```python
from build123d import *

# Parameters (mm, degrees)
SKETCH_1_R          = 1
EXTRUDE_1_DEPTH     = 3
FILLET_1_R          = 10
FILLET_2_R          = 10
FILLET_3_R          = 5
FILLET_4_R          = 3
FILLET_5_R          = 10
SKETCH_5_R          = 1.5
CUT_EXTRUDE_2_DEPTH = 10
SKETCH_6_W          = 40
SKETCH_6_H          = 36.981974808
CUT_EXTRUDE_3_DEPTH = 10
FILLET_6_R          = 10
SKETCH_7_R          = 1.5
CUT_EXTRUDE_4_DEPTH = 31


with BuildPart() as part:
    # Sketch 1 → Extrude 1 (new body)
    with BuildSketch(Plane.XY):
        Polygon((0, -15), (0, 15), (41, 15), (49, 67.5), (180.2, 67.5), (180.2, 49.5), (68.511096619, 49.5), (60.968239476, 0), (68.511096619, -49.5), (180.2, -49.5), (180.2, -67.5), (49, -67.5), (41, -15), align=None)
        with Locations((177.2, 54)):
            Circle(SKETCH_1_R, mode=Mode.SUBTRACT)
        with Locations((177.2, 63)):
            Circle(SKETCH_1_R, mode=Mode.SUBTRACT)
        with Locations((177.2, -54)):
            Circle(SKETCH_1_R, mode=Mode.SUBTRACT)
        with Locations((177.2, -63)):
            Circle(SKETCH_1_R, mode=Mode.SUBTRACT)
        with Locations((71, 58.5)):
            Circle(SKETCH_1_R, mode=Mode.SUBTRACT)
        with Locations((54, 58.5)):
            Circle(SKETCH_1_R, mode=Mode.SUBTRACT)
        with Locations((71, -58.5)):
            Circle(SKETCH_1_R, mode=Mode.SUBTRACT)
        with Locations((54, -58.5)):
            Circle(SKETCH_1_R, mode=Mode.SUBTRACT)
        with BuildLine():
            Line((85, -56), (97, -56))
            ThreePointArc((97, -56), (99.5, -58.5), (97, -61))
            Line((97, -61), (85, -61))
            ThreePointArc((85, -61), (82.5, -58.5), (85, -56))
        make_face(mode=Mode.SUBTRACT)
        with BuildLine():
            Line((85, 56), (97, 56))
            ThreePointArc((97, 56), (99.5, 58.5), (97, 61))
            Line((97, 61), (85, 61))
            ThreePointArc((85, 61), (82.5, 58.5), (85, 56))
        make_face(mode=Mode.SUBTRACT)
    extrude(amount=EXTRUDE_1_DEPTH)

    # Fillet 1
    fillet_1_edges = [part.edges().sort_by_distance(p)[0] for p in [
        (41, -15, 1.5),
        (41, 15, 1.5),
    ]]
    fillet(fillet_1_edges, radius=FILLET_1_R)

    # Fillet 2
    fillet_2_edges = [part.edges().sort_by_distance(p)[0] for p in [
        (68.511096619, -49.5, 1.5),
        (68.511096619, 49.5, 1.5),
    ]]
    fillet(fillet_2_edges, radius=FILLET_2_R)

    # Fillet 3
    fillet_3_edges = [part.edges().sort_by_distance(p)[0] for p in [
        (0, -15, 1.5),
        (0, 15, 1.5),
    ]]
    fillet(fillet_3_edges, radius=FILLET_3_R)

    # Fillet 4
    fillet_4_edges = [part.edges().sort_by_distance(p)[0] for p in [
        (180.2, -49.5, 1.5),
        (180.2, -67.5, 1.5),
        (49, -67.5, 1.5),
        (49, 67.5, 1.5),
        (180.2, 67.5, 1.5),
        (180.2, 49.5, 1.5),
    ]]
    fillet(fillet_4_edges, radius=FILLET_4_R)

    # Fillet 5
    fillet_5_edges = [part.edges().sort_by_distance(p)[0] for p in [
        (60.968239476, 0, 1.5),
    ]]
    fillet(fillet_5_edges, radius=FILLET_5_R)

    # Sketch 5 → Cut-Extrude 2 (cut)
    with BuildSketch(Plane.XY.offset(3)):
        with Locations((134.2, 63)):
            Circle(SKETCH_5_R)
    extrude(amount=-CUT_EXTRUDE_2_DEPTH, mode=Mode.SUBTRACT)

    # Sketch 6 → Cut-Extrude 3 (cut)
    with BuildSketch(Plane.XY.offset(3)):
        with Locations((20, 0)):
            Rectangle(SKETCH_6_W, SKETCH_6_H)
    extrude(amount=-CUT_EXTRUDE_3_DEPTH, mode=Mode.SUBTRACT)

    # Fillet 6
    fillet_6_edges = [part.edges().sort_by_distance(p)[0] for p in [
        (40, 18.490987404, 1.5),
        (40, -18.490987404, 1.5),
    ]]
    fillet(fillet_6_edges, radius=FILLET_6_R)

    # Sketch 7 → Cut-Extrude 4 (cut)
    with BuildSketch(Plane.XY.offset(3)):
        with Locations((44, 9)):
            Circle(SKETCH_7_R)
        with Locations((56, 9)):
            Circle(SKETCH_7_R)
        with Locations((44, -9)):
            Circle(SKETCH_7_R)
        with Locations((56, -9)):
            Circle(SKETCH_7_R)
    extrude(amount=-CUT_EXTRUDE_4_DEPTH, mode=Mode.SUBTRACT)


solid = part.part
```
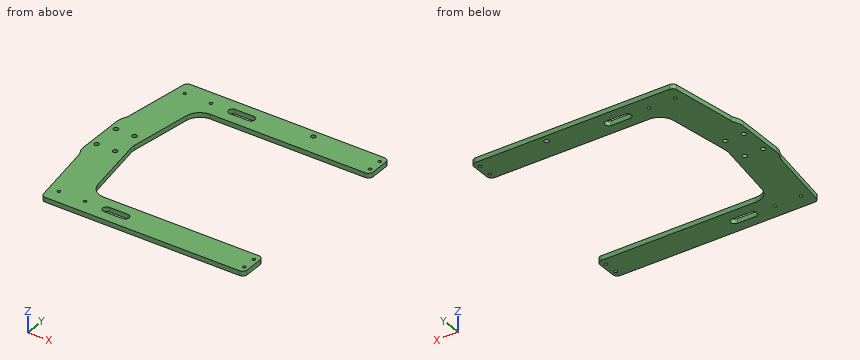
Geometry check sheet. Reference: the model listing, model coordinates, mm. Give positions to 0.01 mm unless a question says otherwise; leave off trailing zeros. Order: outer loops, then holes, each group sorted by start corner. A loop starts at its lowest first (then second) coordinate and runs counter-clockwise, first axis right, second up.
1. Thickness scan on L1, parallel to Y at x = 177.2, z = 2; L2, parallel to Y at x = 96, z = 1.95; L3, parallel to Y at x = 54, z = 1.45. Record the ranges inside material, lowest first.
2. Section check D-D, the plane y = -5.5. Enter the section's corners in (x, z).
3. Gauge pin test, flat ends, axial feed: pin 1 Ø1.6 at (x, y) = (71, -58.5) entering from +Z; pin 2 Ø1 at (y, z) = (-43, 2) entering from -X. Record the tip position at first contact, or that the pin passes through.
4. Section check C-C, the plane y = 26.5. Enter the section's corners in (x, z).
5. Section check B-B, the plane z = 1.45. Give the number of separate pieces and of enclosed holes in the cut face, and give its area (3 significant figures).
6. Section check A-A, the plane x = 121. Enter the section's corners in (y, z), and give its area (3 significant figures).
Values follow:
1. L1: y = -67.5 to -64, -62 to -55, -53 to -49.5, 49.5 to 53, 55 to 62, 64 to 67.5
1. L2: y = -67.5 to -61, -56 to -49.5, 49.5 to 56, 61 to 67.5
1. L3: y = -67.5 to -59.5, -57.5 to 57.5, 59.5 to 67.5
2. outline: (40, 0) - (61.81, 0) - (61.81, 3) - (40, 3) - close
3. pin 1: passes through
3. pin 2: stops at x = 45.19
4. outline: (42.75, 0) - (65.01, 0) - (65.01, 3) - (42.75, 3) - close
5. separate pieces: 1
5. enclosed holes: 15
5. area: 6,780 mm2
6. outline: (-67.5, 0) - (-49.5, 0) - (-49.5, 3) - (-67.5, 3) - close; (49.5, 0) - (67.5, 0) - (67.5, 3) - (49.5, 3) - close
6. area: 108 mm2
